Geometry check sheet. Reference: the model listing, model coordinates, mm. A direction names the side the tool comes from. Give positions to 0.01 mm unless a question says otherwise; leave off trailing zeros. Loops run counter-clockwise (first coordinate to the right, second up) from the corner with the lowest first, then second, coordinate; pieces in that order, holes last. Notation, with made-up numbers: (23.5, 10.25) - (57.5, 10.25) arc R4 ccw to (57.5, 15.25) - close; hole circle Ø7 at (-36.5, 84). An arc over 180 degrees is marked (long way). Use a Markdown table: item, result. Add a question column.
1. Cross-section at B-B on x = 18. Enter the section's corners in (y, z), and give its area (3 significant figures).
2. Set-up check for faces 1 (the flat face through (-27.94, 3, 2)), 2 (the cylindrical face through (-13.15, 0.57, 0.49)), 3 (the flat face through (-21, 3, 4)): record each of +Z, -Z, +X, -X, +Y, -Y from which the full face is reachable in a straight line by a thin tool's end or side.
3. Cross-section at C-C on z = -19. Enter the section's corners in (x, y).
4. Material ranges on L1, parallel to Y at x = 24.13, z = 0.6 (3 decimals); L2, parallel to X at y = 2.5, z = 2.5; L3, parallel to Z at x = -16, y = 4, recorded low to high.
5. Draft check along X on faces 4 (the flat face through (-20, 3, 1)), 5 (the flat face through (21, 3, 4)), 6 (the flat face through (35.13, -2, -11)). Enter one of: pulls with the +X half, pulls with the -X half, needs draft (parallel to the pull), parting line crosses it, or undercut.
6. Depth check by flat-ended pin: P1, Ø3.5, axis at x = 24.13, y = 3.175, coming from the +Z side; P2, Ø4.5, axis at y = 3.5, z = 3, coming from the +X side; P3, Ø3, axis at x = -24, y = 4.5, coming from the -Z side. Enter the tip coordinate at first touch or a pass-through.
7. Cross-section at A-A on x = -24.13. Enter the section's corners in (y, z) (3 decimals), and give its area (3 significant figures).
8. Cross-section at D-D on x = -9. Enter the section's corners in (y, z), and give its area (3 significant figures).
Autodesk Inventor part; units mm, degrees
ref_plane "YZ Plane" through (0, 0, 0) normal (1, 0, 0) x (0, 1, 0)
ref_plane "XZ Plane" through (0, 0, 0) normal (0, 1, 0) x (-1, 0, 0)
ref_plane "XY Plane" through (0, 0, 0) normal (0, 0, 1) x (1, 0, 0)
sketch "Sketch1" plane through (0, 0, 0) normal (0, 0, 1) x (1, 0, 0)
  circle A0 centre (-24.13, 3.175) radius 1.6
  circle A1 centre (24.13, 3.175) radius 1.6
  line L0 (-30.13, 0) -> (30.13, 0)
  line L1 (30.13, 0) -> (30.13, 6.35)
  line L2 (30.13, 6.35) -> (-30.13, 6.35)
  line L3 (-30.13, 6.35) -> (-30.13, 0)
  line L4 (24.13, 3.175) -> (-24.13, 3.175) construction
  line L5 (-24.13, 3.175) -> (0, 0) construction
  line L6 (0, 0) -> (24.13, 3.175) construction
  line L7 (-30.13, 0) -> (-24.13, 3.175) construction
  line L8 (-30.13, 6.35) -> (-24.13, 3.175) construction
  line L9 (24.13, 3.175) -> (30.13, 6.35) construction
  dimension "d0" = 3.2
  dimension "d1" = 48.26
  dimension "d2" = 6
  dimension "d22" = 6.35
extrude "Extrusion1" add sketch "Sketch1" along normal blind 4
sketch "Sketch2" plane through (-30.13, 6.35, 0) normal (0, 1, 0) x (1, 0, 0)
  line L0 (2.19, -3) -> (58.07, -3)
  line L1 (58.07, -3) -> (58.07, -1)
  line L2 (58.07, -1) -> (2.19, -1)
  line L3 (2.19, -1) -> (2.19, -3)
  line L4 (58.07, -1) -> (60.26, 0) construction
  line L5 (0, -4) -> (60.26, -4) construction
  line L6 (58.07, -3) -> (60.26, -4) construction
  line L7 (0, -4) -> (2.19, -3) construction
  point P0 (30.13, 0)
  dimension "d6" = 55.88
  dimension "d7" = 2
extrude "Extrusion2" cut sketch "Sketch2" against normal blind 6.35
sketch "Sketch4" plane through (0, 0, 4) normal (0, 0, 1) x (1, 0, 0)
  line L0 (30.13, 6.35) -> (-30.13, 6.35)
  line L1 (-30.13, 0) -> (30.13, 0)
  line L2 (-13.75, 6.35) -> (13.75, 6.35)
  line L3 (13.75, 6.35) -> (13.75, 0)
  line L4 (13.75, 0) -> (-13.75, 0)
  line L5 (-13.75, 0) -> (-13.75, 6.35)
  line L6 (13.75, 6.35) -> (0, 0) construction
  line L7 (-13.75, 6.35) -> (0, 0) construction
  dimension "d18" = 27.5
extrude "Extrusion4" cut sketch "Sketch4" against normal through all
sketch "Sketch3" plane through (-30.13, 0, 0) normal (0, -1, 0) x (1, 0, 0)
  line L0 (65.26, 9) -> (-5, 9)
  line L1 (-5, 9) -> (-5, -31)
  line L2 (-5, -31) -> (65.26, -31)
  line L3 (65.26, -31) -> (65.26, 9)
  line L4 (0, 4) -> (60.26, 4) construction
  line L5 (0, 4) -> (-5, 9) construction
  line L6 (60.26, 4) -> (65.26, 9) construction
  line L7 (16.88, -6.75) -> (43.38, -6.75)
  line L8 (43.38, -6.75) -> (43.38, -24.25)
  line L9 (43.38, -24.25) -> (16.88, -24.25)
  line L10 (16.88, -24.25) -> (16.88, -6.75)
  line L11 (43.38, -6.75) -> (60.26, 0) construction
  line L12 (43.38, -24.25) -> (65.26, -31) construction
  line L13 (16.88, -6.75) -> (0, 0) construction
  line L14 (16.88, -24.25) -> (-5, -31) construction
  line L15 (16.88, -6.75) -> (16.88, 0) construction
  line L16 (16.88, -24.25) -> (16.88, -31) construction
  line L17 (16.38, 0) -> (0, 0) construction
  point P0 (30.13, 0)
  dimension "d12" = 5
  dimension "d13" = 5
  dimension "d14" = 40
  dimension "d23" = 17.5
  dimension "d24" = 26.5
extrude "Extrusion3" add sketch "Sketch3" along normal blind 5 contours L3 L2 L1 L0 | L7 L8 L9 L10
extrude "Extrusion5" cut sketch "Sketch3" along normal blind 3 contours L7 L8 L9 L10
fillet "Fillet1" radius 2 12 edges at (-13.75, 6.35, 3.5) (-13.75, 6.35, 0.5) (-13.75, 0, 0.5) (-13.75, 0, 3.5) (13.75, 0, 3.5) (13.75, 0, 0.5) (13.75, 6.35, 3.5) (13.75, 6.35, 0.5) (13.25, 0, -15.5) (0, 0, -24.25) (-13.25, 0, -15.5) (0, 0, -6.75)
properties part number "Holder"
Values found:
| question | item | result |
|---|---|---|
| 1 | outline | (-5, -31) - (0, -31) - (0, 0) - (6.35, 0) - (6.35, 1) - (0, 1) - (0, 3) - (6.35, 3) - (6.35, 4) - (0, 4) - (0, 9) - (-5, 9) - close |
| 1 | area | 213 mm2 |
| 2 | face 1 | +Y |
| 2 | face 2 | +Z, -Z, +Y |
| 2 | face 3 | +Z, +X, -X, +Y |
| 3 | outline | (-35.13, -5) - (35.13, -5) - (35.13, 0) - (15.25, 0) arc R2 ccw to (13.25, -2) - (13.25, -3) - (-13.25, -3) - (-13.25, -2) arc R2 ccw to (-15.25, 0) - (-35.13, 0) - close |
| 4 | L1 | y = -5 to 1.575, 4.775 to 6.35 |
| 4 | L2 | x = -30.13 to -27.94, 27.94 to 30.13 |
| 4 | L3 | z = 0 to 1, 3 to 4 |
| 5 | face 4 | undercut |
| 5 | face 5 | needs draft |
| 5 | face 6 | pulls with the +X half |
| 6 | P1 | stops at z = 4 |
| 6 | P2 | stops at x = 30.13 |
| 6 | P3 | stops at z = 0 |
| 7 | outline | (-5, -31) - (0, -31) - (0, 0) - (1.575, 0) - (1.575, 1) - (0, 1) - (0, 3) - (1.575, 3) - (1.575, 4) - (0, 4) - (0, 9) - (-5, 9) - close; (4.775, 0) - (6.35, 0) - (6.35, 1) - (4.775, 1) - close; (4.775, 3) - (6.35, 3) - (6.35, 4) - (4.775, 4) - close |
| 7 | area | 206 mm2 |
| 8 | outline | (-5, -31) - (0, -31) - (0, -26.25) arc R2 ccw to (-2, -24.25) - (-3, -24.25) - (-3, -6.75) - (-2, -6.75) arc R2 ccw to (0, -4.75) - (0, 9) - (-5, 9) - close |
| 8 | area | 146 mm2 |
